```python
from build123d import *

# Parameters (mm, degrees)
F1_DEPTH = 5.5
F2_R     = 8
F3_DEPTH = 1
F4_R     = 3
F5_DEPTH = 30


with BuildPart() as f1:
    # F0 (on Front) → F1 (new body)
    with BuildSketch(Plane.XZ):
        Polygon((0, 5), (2.886751, 0), (8.660254, 0), (11.547005, 5), (8.660254, 10), (2.886751, 10), align=None)
    extrude(amount=F1_DEPTH)

    # F2 (on face) → F3 (join)
    with BuildSketch(Plane(origin=(0, 0, 0), x_dir=(-1, 0, 0), z_dir=(0, 1, 0))):
        with Locations((-5.773503, 5)):
            Circle(F2_R)
        Polygon((-2.886751, 10), (0, 5), (-2.886751, 0), (-8.660254, 0), (-11.547005, 5), (-8.660254, 10), align=None, mode=Mode.SUBTRACT)
    extrude(amount=-F3_DEPTH)

    # F4 (on face) → F5 (join)
    with BuildSketch(Plane(origin=(0, 0, 0), x_dir=(-1, 0, 0), z_dir=(0, 1, 0))):
        with Locations((-5.773503, 5)):
            Circle(F4_R)
    extrude(amount=F5_DEPTH)


solid = f1.part
```
The model under review builds one solid part; all positions refer to its coordinate system, in mm. A direction names the side the tool comes from. Give positions to 0.01 mm unless a question says otherwise; leave off trailing zeros. Write each loop counter-clockwise with the first axis right and the second up, starting at its lowest first coordinate (ties: lowest second). Pieces come first, ordered by that corner, then holes. Notation, with made-up numbers: M -9,-28.75 L 36,-28.75 A19 ccw 36,-13.75 Z; hole C 79.25,-32.75 d9. An arc over 180 degrees is marked long. Answer in a Markdown table with one row per item.
Item 1: Add section A-A on x = 4. Give the boundary of the cut face in (y, z).
Check sheet entries:
| item | result |
|---|---|
| outline | M -5.5,0 L -1,0 L -1,-2.8 L 0,-2.8 L 0,2.58 L 30,2.58 L 30,7.42 L 0,7.42 L 0,12.8 L -1,12.8 L -1,10 L -5.5,10 Z |
Item 2: For line 1 along Y through (x, z) = (10.25, 11.25); line 2 along Y through (x, z) = (2.25, 7.5); line 3 along Z through (x, y) = (11, -2), list the stretches that pass through material, from the lowest coordinate up.
Check sheet entries:
| item | result |
|---|---|
| line 1 | -1 to 0 |
| line 2 | -5.5 to 0 |
| line 3 | 4.05 to 5.95 |
Item 3: Add section B-B on z = 4.25. Give the boundary of the cut face in (x, y), plus the area to 3 significant figures.
Check sheet entries:
| item | result |
|---|---|
| outline | M -2.19,-1 L 0.43,-1 L 0.43,-5.5 L 11.11,-5.5 L 11.11,-1 L 13.74,-1 L 13.74,0 L 8.68,0 L 8.68,30 L 2.87,30 L 2.87,0 L -2.19,0 Z |
| area | 238 mm2 |
Item 4: Tool access review of faces 1 (the face through (5.9, -1, -0.2)), 2 (the face through (6, -3, 0)), 3 (the face through (1.423, -3.218, 2.535)), 4 (the face through (6.42, 14.79, 2.07)), 5 (the face through (6, -3, 10)): name each direction out of +Z, -Z, +X, -X, +Y, -Y from which nothing blocks a thin tool from reaching the whole face with its end or side.
Check sheet entries:
| item | result |
|---|---|
| face 1 | -Y |
| face 2 | -Z, +X, -X, -Y |
| face 3 | -Z, -X, -Y |
| face 4 | +Y |
| face 5 | +Z, +X, -X, -Y |
Item 5: Add section D-D on z = -0.75. Give the boundary of the cut face in (x, y).
Check sheet entries:
| item | result |
|---|---|
| outline | M 0.21,-1 L 11.34,-1 L 11.34,0 L 0.21,0 Z |
Item 6: Add section C-C on y = 10. Give the boundary of the cut face in (x, z), plus the area to 3 significant figures.
Check sheet entries:
| item | result |
|---|---|
| outline | C 5.77,5 d6 |
| area | 28.3 mm2 |
Item 7: For P1, Ø8, axis at y = 17.5, z = 11.5, coming from the +X side; P2, Ø5, axis at x = 8.5, y = 20.5, coming from the -Z side; P3, Ø5, axis at y = 7, z = 6.5, coming from the -X side, all flat-tipped, find the tip position at first contact; note any pin that passes through.
Check sheet entries:
| item | result |
|---|---|
| P1 | x = 7.43 |
| P2 | z = 2.01 |
| P3 | x = 2.77 |
